from build123d import *

# Parameters (mm, degrees)
SKETCH5_W                 = 11.25
SKETCH5_H                 = 8.5
EXTRUDE4_DEPTH            = 2.5
SKETCH19_W                = 1.5
SKETCH19_H                = 8.5
EXTRUDE12_DEPTH           = 1.5
SKETCH21_W                = 9
SKETCH21_H                = 7
EXTRUDE13_DEPTH           = 3.5
SKETCH22_W                = 4
SKETCH22_H                = 2.302396537
EXTRUDE14_DEPTH           = 3.75
EXTRUDE15_DEPTH           = 0.75
EXTRUDE18_DEPTH           = 13.25
F_0_80_TAPPED_HOLE1_D     = 1.19126
F_0_80_TAPPED_HOLE1_DEPTH = 79.01
F_0_80_TAPPED_HOLE1_TIP   = 0.357890611
FILLET4_R                 = 1


with BuildPart() as part:
    # Sketch5 → Extrude4 (new body)
    with BuildSketch(Plane(origin=(0, 0, 0), x_dir=(1, 0, 0), z_dir=(0, 1, 0))):
        Rectangle(SKETCH5_W, SKETCH5_H)
    extrude(amount=EXTRUDE4_DEPTH)

    # Sketch19 → Extrude12 (cut)
    with BuildSketch(Plane(origin=(0, 2.5, 0), x_dir=(-1, 0, 0), z_dir=(0, 1, 0))):
        with Locations((4.875, 0)):
            Rectangle(SKETCH19_W, SKETCH19_H)
    extrude(amount=-EXTRUDE12_DEPTH, mode=Mode.SUBTRACT)

    # Sketch21 → Extrude13 (cut, through all)
    with BuildSketch(Plane(origin=(0, 2.5, 0), x_dir=(-1, 0, 0), z_dir=(0, 1, 0))):
        with Locations((-0.375, 0)):
            Rectangle(SKETCH21_W, SKETCH21_H)
    extrude(amount=-EXTRUDE13_DEPTH, mode=Mode.SUBTRACT)

    # Sketch22 → Extrude14 (add)
    with BuildSketch(Plane.XY.offset(4.25)):
        with Locations((-0.875, 1.348801732)):
            Rectangle(SKETCH22_W, SKETCH22_H)
    extrude(amount=EXTRUDE14_DEPTH)

    # Sketch24 → Extrude15 (add)
    with BuildSketch(Plane(origin=(0, 2.5, 0), x_dir=(1, 0, 0), z_dir=(0, 1, 0))):
        Polygon((-4.125, 3.85), (-4.125, 3.5), (4.875, 3.5), (4.875, -3.5), (-4.125, -3.5), (-4.125, -3.85), (5.225, -3.85), (5.225, 3.85), align=None)
    extrude(amount=EXTRUDE15_DEPTH)

    # Sketch33 → Extrude18 (cut, through all)
    with BuildSketch(Plane(origin=(0, 0, -4.25), x_dir=(-1, 0, 0), z_dir=(0, 0, -1))):
        with BuildLine():
            Line((38.114202873, -7.832830513), (5.625, 0))
            ThreePointArc((5.625, 0), (0, 0.668489655), (-5.625, 0))
            Line((-5.625, 0), (-38.114202873, -7.832830513))
            Line((-38.114202873, -7.832830513), (-38.114202873, -74.672984228))
            Line((-38.114202873, -74.672984228), (38.114202873, -74.672984228))
            Line((38.114202873, -74.672984228), (38.114202873, -7.832830513))
        make_face()
    extrude(amount=-EXTRUDE18_DEPTH, mode=Mode.SUBTRACT)

    # #0-80 Tapped Hole1
    with Locations(Plane(origin=(-0.875, 2.5, 6), x_dir=(0, 0, 1), z_dir=(0, 1, 0))):
        with Locations((0, 0)):
            Hole(F_0_80_TAPPED_HOLE1_D / 2, depth=F_0_80_TAPPED_HOLE1_DEPTH)
            with Locations((0, 0, -(F_0_80_TAPPED_HOLE1_DEPTH + F_0_80_TAPPED_HOLE1_TIP / 2))):  # 118° drill point
                Cone(0, F_0_80_TAPPED_HOLE1_D / 2, F_0_80_TAPPED_HOLE1_TIP, mode=Mode.SUBTRACT)

    # Fillet4
    fillet4_edges = [part.edges().sort_by_distance(p)[0] for p in [
        (5.625, 1.25, -4.25),
        (5.225, 2.875, -3.85),
        (5.625, 1.25, 4.25),
        (5.225, 2.875, 3.85),
        (4.875, 1.709078603, 3.5),
        (4.875, 1.709078603, -3.5),
        (-4.125, 0.655670027, 3.5),
        (-4.125, 0.655670027, -3.5),
        (-5.625, 0.5, -4.25),
        (-5.625, 0.5, 4.25),
        (-2.875, 1.497833445, 4.25),
        (-2.875, 1.497833445, 8),
        (1.125, 1.571053984, 8),
        (1.125, 1.571053984, 4.25),
    ]]
    fillet(fillet4_edges, radius=FILLET4_R)


solid = part.part
The listing builds one solid part. Answer for the finished solid, in the listing's coordinates (mm). A direction names the side the tool comes from. Give positions to 0.01 mm unless a question says otherwise; leave off trailing zeros. Order: outer loops, then holes, each group sorted by start corner. A loop starts at its lowest first (then second) coordinate and runs counter-clockwise, first axis right, second up. Notation, with made-up numbers: (-29.5, -1) -> (26.5, -1) arc R13 ccw to (26.5, 18) -> close; hole circle Ø3 at (13.25, -10.75). An arc over 180 degrees is marked (long way). Put each result on its own line as item: value.
Item 1: Given P1, Ø1.1, axis at x = 3, y = 2, coming from the +Z side; P2, Ø5, axis at x = -0.5, z = 6, coming from the -Y side; P3, Ø1.5, axis at x = -0.875, z = 6, coming from the +Y side; P4, Ø5, axis at x = -3.5, z = 2.5, coming from the -Y side, each flat-ended and moving along its own axis, determine where each tip first touches the part or whether it passes through.
Established:
P1: stops at z = 4.25
P2: stops at y = 0.5
P3: stops at y = 2.5
P4: stops at y = 0
Item 2: For faces 1 (the face through (3, 1, 4.25)), 2 (the face through (-5.324, 0.507, -3.965)), 3 (the face through (0, 2.5, 4.1)), 4 (the face through (-2.875, 1, 6)), determine the directions among +Z, -Z, +X, -X, +Y, -Y from which every point of the face is accessible in a straight line to the end or side of a thin tool.
Established:
face 1: +Z, +X, +Y, -Y
face 2: -Z, -X, +Y, -Y
face 3: +X, +Y
face 4: +Z, -X, +Y, -Y
Item 3: For a pull along X with two mould halves and no side action, classify faces 5 (the face through (5.03, 3.25, -0.02)), 6 (the face through (4.875, 2, 0)), 7 (the face through (4.924, 2.88, -3.565)), 8 (the face through (4.59, 1.73, 3.2)) as released by +X, released by -X, zero draft, split by the parting line, or undercut.
Established:
face 5: zero draft
face 6: undercut
face 7: released by +X
face 8: undercut
Item 4: A cutting plane is placed at D-D on z = 6. Give the vertices of the cut face in (x, y) (3 decimals).
Established:
outline: (-2.875, 0.496) arc R24 cw to (-1.471, 0.623) -> (-1.471, 2.5) -> (-2.875, 2.5) -> close; (-0.279, 0.667) arc R24 cw to (1.125, 0.642) -> (1.125, 2.5) -> (-0.279, 2.5) -> close
Item 5: A cutting plane is placed at C-C on y = 2.9. Give the vertices of the cut face in (x, z) (3 decimals), plus the area to 4 significant figures.
Established:
outline: (-4.125, -3.85) -> (4.225, -3.85) arc R1 ccw to (5.225, -2.85) -> (5.225, 2.85) arc R1 ccw to (4.225, 3.85) -> (-4.125, 3.85) -> (-4.125, 3.5) -> (3.875, 3.5) arc R1 cw to (4.875, 2.5) -> (4.875, -2.5) arc R1 cw to (3.875, -3.5) -> (-4.125, -3.5) -> close
area: 8.995 mm^2
Item 6: A cutting plane is placed at B-B on x = -1.25. Give the vertices of the cut face in (y, z), plus the area to 3 significant figures.
Established:
outline: (0.64, -4.25) -> (2.5, -4.25) -> (2.5, -3.85) -> (3.25, -3.85) -> (3.25, -3.5) -> (0.64, -3.5) -> close; (0.64, 3.5) -> (3.25, 3.5) -> (3.25, 3.85) -> (2.5, 3.85) -> (2.5, 5.54) -> (0.64, 5.54) -> close; (0.64, 6.46) -> (2.5, 6.46) -> (2.5, 8) -> (0.64, 8) -> close
area: 8.59 mm^2
Item 7: A cutting plane is placed at A-A on z = -0.5. Give the vertices of the cut face in (x, y) (3 decimals), plus the area to 3 significant figures.
Established:
outline: (-5.625, 0) arc R24 cw to (-4.125, 0.311) -> (-4.125, 1) -> (-5.625, 1) -> close; (4.875, 0.168) arc R24 cw to (5.625, 0) -> (5.625, 2.5) -> (5.225, 2.5) -> (5.225, 3.25) -> (4.875, 3.25) -> close
area: 3.33 mm^2
Item 8: Straight lines are drawn through the part: line 1 (Z direction, x = 3.5, y = 0.5); line 2 (Z direction, x = -1.75, y = 1.95); line 3 (X direction, y = 2.1, z = 6) (3 decimals). For each, find the intervals that lie inside material, in ascending order.
Established:
line 1: z = -4.25 to -3.5, 3.5 to 4.25
line 2: z = -4.25 to -3.5, 3.5 to 8
line 3: x = -2.875 to -1.471, -0.279 to 1.125
